Read the model definition and answer for the solid it produces. Units are mm, in the model's axes. A direction names the side the tool comes from. Give positions to 0.01 mm unless a question says otherwise; leave off trailing zeros. Loops run counter-clockwise (first coordinate to the right, second up) from the corner with the lowest first, then second, coordinate; pieces in that order, holes last. Notation, with made-up numbers: (-8.5, 61) -> (0.5, 61) arc R32 ccw to (0.5, 98) -> close; hole circle Ø11 at (79, -13.5). An arc over 180 degrees is marked (long way). Return JSON: item names as keys, results as strings. Group by question number.
from build123d import *

# Parameters (mm, degrees)
F0_W          = 90
F0_H          = 30
F0_R          = 6
F1_DEPTH      = 20
F2_SIZE       = 1
F3_R          = 9.5
F4_DEPTH      = 5
F4_DEPTH_BACK = 38
F5_SIZE       = 1
F6_T4_ANGLE   = 359.64
F6_S5_R       = 6
F6_T6_DEPTH   = 29
F6_S7_R       = 6
F6_T8_DEPTH   = 29
F6_T12_ANGLE  = 359.64
F6_S13_R      = 6
F6_T14_DEPTH  = 29
F6_S15_R      = 6
F6_T16_DEPTH  = 29


# Not quite as in the source:
# - a fillet or chamfer that OpenCascade refuses, or shapes differently, is made with other operations: its cross-section is extruded or revolved along the edge and cut away or added


with BuildPart() as f1:
    # F0 (on Top) → F1 (new body)
    with BuildSketch(Plane.XY):
        Rectangle(F0_W, F0_H)
        with Locations((-30, 0)):
            Circle(F0_R, mode=Mode.SUBTRACT)
        with Locations((-10, 0)):
            Circle(F0_R, mode=Mode.SUBTRACT)
        with Locations((10, 0)):
            Circle(F0_R, mode=Mode.SUBTRACT)
        with Locations((30, 0)):
            Circle(F0_R, mode=Mode.SUBTRACT)
    extrude(amount=F1_DEPTH)

    # F2
    f2_edges = [f1.edges().sort_by_distance(p)[0] for p in [
        (0, 15, 20),
        (-45, 0, 20),
        (0, -15, 20),
        (45, 0, 20),
        (-36, 0, 20),
        (-16, 0, 20),
        (4, 0, 20),
        (24, 0, 20),
    ]]
    chamfer(f2_edges, length=F2_SIZE)

    # F3 (on Top) → F4 (join, two sides)
    with BuildSketch(Plane.XY) as f4_sk:
        Circle(F3_R)
    extrude(amount=F4_DEPTH)
    extrude(f4_sk.sketch, amount=-F4_DEPTH_BACK)

    # F5
    f5_edges = [f1.edges().sort_by_distance(p)[0] for p in [
        (-9.5, 0, -38),
    ]]
    chamfer(f5_edges, length=F5_SIZE)

    # F6: fillet of radius 5 on 2 edges, made by hand


with BuildPart() as f6_tool2:
    # F6_s3 → F6_t4 (revolve)
    with BuildSketch(Plane(origin=(0, 0, 0), x_dir=(0, 0, 1), z_dir=(0.9999950652, 0.0031415875, 0))):
        with BuildLine():
            ThreePointArc((-5, -9.5), (-1.4644660941, -10.9644660941), (0, -14.5))
            Line((0, -14.5), (0, -9.5))
            Line((0, -9.5), (-5, -9.5))
        make_face()
    revolve(axis=Axis((0, 0, 0), (0, 0, 1)), revolution_arc=F6_T4_ANGLE)

    # F6_s5 → F6_t6 (cut, symmetric)
    with BuildSketch(Plane.XY.offset(-2.5)):
        with Locations((10, 0)):
            Circle(F6_S5_R)
    extrude(amount=F6_T6_DEPTH, both=True, mode=Mode.SUBTRACT)

    # F6_s7 → F6_t8 (cut, symmetric)
    with BuildSketch(Plane.XY.offset(-2.5)):
        with Locations((-10, 0)):
            Circle(F6_S7_R)
    extrude(amount=F6_T8_DEPTH, both=True, mode=Mode.SUBTRACT)


with BuildPart() as f1_1:
    add(f1.part)

    # F6_t1: union F6_tool2
    add(f6_tool2.part)


with BuildPart() as f6_tool10:
    # F6_s11 → F6_t12 (revolve)
    with BuildSketch(Plane(origin=(0, 0, 0), x_dir=(0, 0, 1), z_dir=(-0.9999950652, -0.0031415875, 0))):
        with BuildLine():
            ThreePointArc((-5, -9.5), (-1.4644660941, -10.9644660941), (0, -14.5))
            Line((0, -14.5), (0, -9.5))
            Line((0, -9.5), (-5, -9.5))
        make_face()
    revolve(axis=Axis((0, 0, 0), (0, 0, 1)), revolution_arc=F6_T12_ANGLE)

    # F6_s13 → F6_t14 (cut, symmetric)
    with BuildSketch(Plane.XY.offset(-2.5)):
        with Locations((10, 0)):
            Circle(F6_S13_R)
    extrude(amount=F6_T14_DEPTH, both=True, mode=Mode.SUBTRACT)

    # F6_s15 → F6_t16 (cut, symmetric)
    with BuildSketch(Plane.XY.offset(-2.5)):
        with Locations((-10, 0)):
            Circle(F6_S15_R)
    extrude(amount=F6_T16_DEPTH, both=True, mode=Mode.SUBTRACT)


with BuildPart() as f1_2:
    add(f1_1.part)

    # F6_t9: union F6_tool10
    add(f6_tool10.part)


solid = f1_2.part
1. Flat-ended cylindrical pins translate along their axes: pin 1 Ø3 at (y, z) = (-0.5, -30) entering from -X; pin 2 Ø4.5 at (x, y) = (-8, 2.5) entering from +Z; pin 3 Ø15.5 at (x, y) = (30, 0) entering from -Z. Find the tip coordinate at first contact, or state that the pin passes through.
2. Section D-D on z = -31 is taken. Determine the outline of the cut face in (x, y).
3. Which of the six approach directions +Z, -Z, +X, -X, +Y, -Y give full straight-line access (tool end or side, diameter ignored) to faces 1 (the flat face through (7, 0, 5)), 2 (the cylindrical face through (9.326, 1.808, -15.706)), 3 (the flat face through (-1, 15, 9))?
4. Section B-B on z = 7.5 is taken. Determine the outline of the cut face in (x, y), then the cut area to 3 significant figures.
5. Section A-A on x = -30 is taken. Determine the outline of the cut face in (y, z), then the cut area to 3 significant figures.
6. Straight lines are drawn through the part: line 1 (X direction, y = 5.5, z = 7.5); line 2 (Y direction, x = 30, z = 11.5); line 3 (X direction, y = -2.5, z = 1). For each, find the intervals that lie inside material, in ascending order. Write a range as from..to.
7. Determine the mould class of faces 4 (the cylindrical face through (24, 0, 9)), 5 (the flat face through (0, 0, -38)), 6 (the flat face through (45, 0, 9)) for opening direction X: pulls with the +X half, pulls with the -X half, needs draft (parallel to the pull), parting line crosses it, or undercut.
8. Section C-C on x = 0 is taken. Determine the outline of the cut face in (y, z), then the cut area to 3 significant figures.
Completed:
{
 "1": {"pin 1": "stops at x = -9.5", "pin 2": "stops at z = 5", "pin 3": "stops at z = 0"},
 "2": {"outline": "circle Ø19 at (0, 0)"},
 "3": {"face 1": "+Z", "face 2": "-Z", "face 3": "+Z, -Z, +X, -X, +Y"},
 "4": {"outline": "(-45, -15) -> (45, -15) -> (45, 15) -> (-45, 15) -> close; hole circle Ø12 at (-30, 0); hole circle Ø12 at (-10, 0); hole circle Ø12 at (10, 0); hole circle Ø12 at (30, 0)", "area": "2,250 mm²"},
 "5": {"outline": "(-15, 0) -> (-6, 0) -> (-6, 19) -> (-7, 20) -> (-14, 20) -> (-15, 19) -> close; (6, 0) -> (15, 0) -> (15, 19) -> (14, 20) -> (7, 20) -> (6, 19) -> close", "area": "358 mm²"},
 "6": {"line 1": "x = -45..-32.4, -27.6..-12.4, -7.6..7.6, 12.4..27.6, 32.4..45", "line 2": "y = -15..-6, 6..15", "line 3": "x = -45..-35.45, -24.55..-15.45, -9.17..9.17, 15.45..24.55, 35.45..45"},
 "7": {"face 4": "undercut", "face 5": "needs draft", "face 6": "pulls with the +X half"},
 "8": {"outline": "(-15, 0) -> (-14.5, 0) arc R5 cw to (-9.5, -5) -> (-9.5, -37) -> (-8.5, -38) -> (8.5, -38) -> (9.5, -37) -> (9.5, -5) arc R5 cw to (14.5, 0) -> (15, 0) -> (15, 19) -> (14, 20) -> (-14, 20) -> (-15, 19) -> close", "area": "1,330 mm²"}
}
